from build123d import *

# Parameters (mm, degrees)
F0_W     = 87.884
F0_H     = 76.2
F1_DEPTH = 43.18
F2_R     = 12.7
F4_DEPTH = 2.54
F5_DEPTH = 2.54
F7_DEPTH = 2.54
F8_R     = 8.636
F9_DEPTH = 76.201


# Not quite as in the source:
# - ends of sketch curves that miss each other by under 0.0002 mm in the source are joined


with BuildPart() as f1:
    # F0 (on Front) → F1 (new body)
    with BuildSketch(Plane.XZ):
        with Locations((43.942, 38.1)):
            Rectangle(F0_W, F0_H)
    extrude(amount=F1_DEPTH)

    # F2
    f2_edges = [f1.edges().sort_by_distance(p)[0] for p in [
        (43.942, -43.18, 76.2),
        (43.942, 0, 76.2),
    ]]
    fillet(f2_edges, radius=F2_R)

    # F3 (on face) → F4 (cut)
    with BuildSketch(Plane.XZ.offset(43.18)):
        Polygon((38.862, 47.2823401565), (43.942, 47.2823401565), (49.022, 47.2823401565), (49.022, 37.1223401565), (59.182, 37.1223401565), (59.182, 26.9623401565), (50.7279873173, 26.9623401565), (85.3440016508, 2.5399983492), (85.3440016508, 60.9600016508), (2.5399983492, 60.9600016508), (36.3272919048, 37.1223401565), (38.862, 37.1223401565), align=None)
    extrude(amount=-F4_DEPTH, mode=Mode.SUBTRACT)

    # F3 (on face) → F5 (cut)
    with BuildSketch(Plane.XZ.offset(43.18)):
        Polygon((50.2873871384, 26.9623401565), (35.8866917258, 37.1223401565), (28.702, 37.1223401565), (28.702, 26.9623401565), (38.862, 26.9623401565), (38.862, 16.8023401565), (43.942, 16.8023401565), (49.022, 16.8023401565), (49.022, 26.9623401565), align=None)
    extrude(amount=-F5_DEPTH, mode=Mode.SUBTRACT)

    # F6 (on face) → F7 (cut)
    with BuildSketch(Plane(origin=(0, 0, 0), x_dir=(-1, 0, 0), z_dir=(0, 1, 0))):
        Polygon((-48.0027233214, 47.2823394346), (-42.9227233214, 47.2823394346), (-37.8427233214, 47.2823394346), (-37.8427233214, 37.1223394346), (-27.6827233214, 37.1223394346), (-27.6827233214, 26.9623394346), (-37.1560138865, 26.9623391642), (-2.54, 2.5399966984), (-2.54, 60.96), (-85.344, 60.96), (-51.5567091082, 37.1223394346), (-48.0027233214, 37.1223394346), align=None)
        Polygon((-37.5966140538, 26.9623391642), (-51.9973092754, 37.1223394346), (-58.1627233214, 37.1223394346), (-58.1627233214, 26.9623394346), (-48.0027233214, 26.9623394346), (-48.0027233214, 16.8023394346), (-42.9227233214, 16.8023394346), (-37.8427233214, 16.8023394346), (-37.8427233214, 26.9623394346), align=None)
    extrude(amount=-F7_DEPTH, mode=Mode.SUBTRACT)

    # F8 (on face) → F9 (cut, through all)
    with BuildSketch(Plane.XY.offset(76.2)):
        with Locations((21.336, -21.59)):
            Circle(F8_R)
        with Locations((66.548, -21.59)):
            Circle(F8_R)
    extrude(amount=-F9_DEPTH, mode=Mode.SUBTRACT)


solid = f1.part
For this review, take the finished solid that the model builds, in its own axes (mm). A direction names the side the tool comes from. Round coordinates to 2 decimals unless told otherwise and drop trailing zeros. Loops run counter-clockwise (first coordinate to the right, second up) from the corner with the lowest first, then second, coordinate; pieces in that order, holes last. Notation, with made-up numbers: (-33, 50.25) - (2, 50.25) arc R34 cw to (2, 83.25) - close; hole circle Ø11 at (34, -6). An arc over 180 degrees is marked (long way). Put each result on its own line as item: value. Start each with the question number.
1. Consider section C-C on z = 28.5. State the section outline as (x, y) points, plus the area to 3 significant figures.
2. For probe 1 along X at (y, z) = (-21, 19); probe 2 along X at (y, z) = (-41, 29.5); probe 3 along Z at (x, y) = (54.5, -31), list the stretches that pass through material, from the lowest coordinate up. Write a range as [from, to].
3. For faces 1 (the flat face through (38.862, -42, 22)), 2 (the flat face through (43, -1, 47.282)), list the 3-axis set-ups (+Z, -Z, +X, -X, +Y, -Y) from which the entire face can be reached by the end or side of a thin tool; tool diameter is ignored.
4. Mouldability with a two-part tool opening along X and no side actions: class faces 3 (the flat face through (87.884, -21, 38)), 4 (the flat face through (38.862, -42, 42)) as +X half, -X half, draft (parallel to the pull), parting line (faces both ways), or undercut.
5. Consider section B-B on x = 15. State the section outline as (y, z) points.
6. Consider section D-D on x = 62.5. State the section outline as (y, z) points, plus the area to 3 significant figures.
7. Insertion check: P1, Ø2, axis at x = 43, y = -41.5, coming from the +Z side; P2, Ø1.3, axis at x = 50.5, y = -1.5, coming from the +Z side; P3, Ø0.8, axis at x = 35, y = -41.5, coming from the +Z side. Each pin has a flat end and moves straight along its axis. Give the tip position at first contact, or say it passes through.
8. Consider section A-A on y = -21.59. State the section outline as (x, z) points, plus the area to 3 significant figures.
Result sheet:
1. outline: (0, -43.18) - (28.7, -43.18) - (28.7, -40.64) - (48.11, -40.64) - (48.11, -43.18) - (59.18, -43.18) - (59.18, -40.64) - (85.34, -40.64) - (85.34, -43.18) - (87.88, -43.18) - (87.88, 0) - (58.16, 0) - (58.16, -2.54) - (39.78, -2.54) - (39.78, 0) - (27.68, 0) - (27.68, -2.54) - (2.54, -2.54) - (2.54, 0) - (0, 0) - close; hole circle Ø17.27 at (21.34, -21.59); hole circle Ø17.27 at (66.55, -21.59)
1. area: 3,100 mm^2
2. probe 1: [0, 12.72], [29.95, 57.93], [75.16, 87.88]
2. probe 2: [0, 28.7], [46.69, 59.18], [85.34, 87.88]
2. probe 3: [0, 76.19]
3. face 1: -Y
3. face 2: +Y
4. face 3: +X half
4. face 4: undercut
5. outline: (-43.18, 0) - (-27.46, 0) - (-27.46, 76.2) - (-30.48, 76.2) arc R12.7 ccw to (-43.18, 63.5) - (-43.18, 60.96) - (-40.64, 60.96) - (-40.64, 52.17) - (-43.18, 52.17) - close; (-15.72, 0) - (0, 0) - (0, 11.33) - (-2.54, 11.33) - (-2.54, 60.96) - (0, 60.96) - (0, 63.5) arc R12.7 ccw to (-12.7, 76.2) - (-15.72, 76.2) - close
6. outline: (-43.18, 0) - (-29.22, 0) - (-29.22, 76.2) - (-30.48, 76.2) arc R12.7 ccw to (-43.18, 63.5) - (-43.18, 60.96) - (-40.64, 60.96) - (-40.64, 18.66) - (-43.18, 18.66) - close; (-13.96, 0) - (0, 0) - (0, 44.84) - (-2.54, 44.84) - (-2.54, 60.96) - (0, 60.96) - (0, 63.5) arc R12.7 ccw to (-12.7, 76.2) - (-13.96, 76.2) - close
6. area: 1,910 mm^2
7. P1: z = 71.3
7. P2: z = 70.57
7. P3: z = 70.46
8. outline: (0, 0) - (12.7, 0) - (12.7, 76.2) - (0, 76.2) - close; (29.97, 0) - (57.91, 0) - (57.91, 76.2) - (29.97, 76.2) - close; (75.18, 0) - (87.88, 0) - (87.88, 76.2) - (75.18, 76.2) - close
8. area: 4,060 mm^2
